Geometry check sheet. Reference: the model listing, model coordinates, mm. A direction names the side the tool comes from. Give positions to 0.01 mm unless a question says otherwise; leave off trailing zeros. Loops run counter-clockwise (first coordinate to the right, second up) from the corner with the lowest first, then second, coordinate; pieces in that order, holes last.
1. Release check for a two-part mould opening along Y. For faces 1 (the cylindrical face through (-1.4, 10.66, 18.24)), 2 (the flat face through (-3.25, -9, 3)), 3 (the flat face through (-1.35, 0, 32)) record: +Y half, -Y half, draft (parallel to the pull), parting line (faces both ways), or undercut.
2. Cross-section at A-A, the plane z = 16.5. Record the cut outline in (x, y).
3. Tool access check on faces 4 (the flat face through (2, 0, 40)), 5 (the flat face through (-2, 0, 25)), 6 (the flat face through (0, -6.5, 32)), 7 (the flat face through (3.25, -9, 3)). Record the directions out of +Z, -Z, +X, -X, +Y, -Y that give a thin tool (end or side, any length) a straight path to the whole face; none if there is none.
4. Go/stop test with flat-tipped pins: pin 1 Ø1 at (x, z) = (-8.5, 28.5) entering from -Y; pin 2 Ø3 at (x, z) = (-8, 6) entering from +Y; pin 3 Ø2.5 at (x, y) = (3, -1.5) entering from -Z. Record where each tip stops, or that it passes through.
5. Cross-section at B-B, the plane z = 4.5. Record the cut outline in (x, y).
6. Material ranges on L1, parallel to X at y = 0, z = 15.75; L2, parallel to Z at x = 2, y = 2.25, recorded low to high.
7. Cross-section at C-C, the plane z = 29. Record the cut outline in (x, y), plus the area to 3 significant figures.
from build123d import *

# Parameters (mm, degrees)
F0_R     = 10.75
F0_R_2   = 7.75
F1_DEPTH = 40
F3_DEPTH = 15
F4_DEPTH = 25
F7_R     = 3
F6_W     = 2.7
F6_H     = 13
F8_DEPTH = 25


# Not quite as in the source:
# - a fillet or chamfer that OpenCascade refuses, or shapes differently, is made with other operations: its cross-section is extruded or revolved along the edge and cut away or added


with BuildPart() as f1:
    # F0 (on Top) → F1 (new body)
    with BuildSketch(Plane.XY):
        Circle(F0_R)
        Circle(F0_R_2, mode=Mode.SUBTRACT)
        Circle(F0_R_2)
    extrude(amount=F1_DEPTH)

    # F2 (on Front) → F3 (cut)
    with BuildSketch(Plane.XZ):
        with BuildLine():
            Line((-3.25, 6), (-3.25, 0))
            Line((-3.25, 0), (3.25, 0))
            Line((3.25, 0), (3.25, 6))
            ThreePointArc((3.25, 6), (0, 9.25), (-3.25, 6))
        make_face()
    extrude(amount=F3_DEPTH, mode=Mode.SUBTRACT)

    # F0 (on Top) → F4 (cut)
    with BuildSketch(Plane.XY):
        Circle(F0_R_2)
    extrude(amount=F4_DEPTH, mode=Mode.SUBTRACT)

    # F7
    f7_edges = [f1.edges().sort_by_distance(p)[0] for p in [
        (-10.75, 0, 40),
    ]]
    fillet(f7_edges, radius=F7_R)

    # F6 (on offset) → F8 (cut)
    with BuildSketch(Plane.XY.offset(40)):
        Rectangle(F6_W, F6_H)
    extrude(amount=-F8_DEPTH, mode=Mode.SUBTRACT)

    # F9: fillet of radius 4 on 1 edges, made by hand


with BuildPart() as f9_tool2:
    # F9_s3 → F9_t4 (revolve)
    with BuildSketch(Plane.XZ):
        with BuildLine():
            ThreePointArc((7.75, 21), (6.5784271247, 23.8284271247), (3.75, 25))
            Line((3.75, 25), (7.75, 25))
            Line((7.75, 25), (7.75, 21))
        make_face()
    revolve(axis=Axis((0, 0, 25), (0, 0, 1)))

    split(bisect_by=Plane.YZ.offset(1.35), keep=Keep.TOP)


with BuildPart() as f1_1:
    add(f1.part)

    # F9_t1: union F9_tool2
    add(f9_tool2.part)


with BuildPart() as f9_tool7:
    # F9_s8 → F9_t9 (revolve)
    with BuildSketch(Plane.XZ):
        with BuildLine():
            ThreePointArc((7.75, 21), (6.5784271247, 23.8284271247), (3.75, 25))
            Line((3.75, 25), (7.75, 25))
            Line((7.75, 25), (7.75, 21))
        make_face()
    revolve(axis=Axis((0, 0, 25), (0, 0, 1)))

    split(bisect_by=Plane.YZ.offset(-1.35), keep=Keep.BOTTOM)


with BuildPart() as f1_2:
    add(f1_1.part)

    # F9_t6: union F9_tool7
    add(f9_tool7.part)


with BuildPart() as f9_tool12:
    # F9_s13 → F9_t14 (revolve)
    with BuildSketch(Plane.XZ):
        with BuildLine():
            ThreePointArc((7.75, 21), (6.5784271247, 23.8284271247), (3.75, 25))
            Line((3.75, 25), (7.75, 25))
            Line((7.75, 25), (7.75, 21))
        make_face()
    revolve(axis=Axis((0, 0, 25), (0, 0, 1)))

    split(bisect_by=Plane.XZ.offset(-6.5), keep=Keep.BOTTOM)


with BuildPart() as f1_3:
    add(f1_2.part)

    # F9_t11: union F9_tool12
    add(f9_tool12.part)


with BuildPart() as f9_tool17:
    # F9_s18 → F9_t19 (revolve)
    with BuildSketch(Plane.XZ):
        with BuildLine():
            ThreePointArc((7.75, 21), (6.5784271247, 23.8284271247), (3.75, 25))
            Line((3.75, 25), (7.75, 25))
            Line((7.75, 25), (7.75, 21))
        make_face()
    revolve(axis=Axis((0, 0, 25), (0, 0, 1)))

    split(bisect_by=Plane.XZ.offset(6.5), keep=Keep.TOP)


with BuildPart() as f1_4:
    add(f1_3.part)

    # F9_t16: union F9_tool17
    add(f9_tool17.part)


solid = f1_4.part
Result:
1. face 1: parting line
1. face 2: draft
1. face 3: undercut
2. outline: circle Ø21.5 at (0, 0); hole circle Ø15.5 at (0, 0)
3. face 4: +Z, +X, -X, +Y, -Y
3. face 5: -Z
3. face 6: +Z, -Z
3. face 7: -Z, -Y
4. pin 1: stops at y = -7.18
4. pin 2: stops at y = 8.56
4. pin 3: stops at z = 24.91
5. outline: (-3.25, -10.25) - (-3.25, -7.04) arc R7.75 cw (long way) to (3.25, -7.04) - (3.25, -10.25) arc R10.75 ccw (long way) to start
6. L1: x = -10.75 to -7.75, 7.75 to 10.75
6. L2: z = 25 to 40
7. outline: circle Ø21.5 at (0, 0); hole (-1.35, -6.5) - (1.35, -6.5) - (1.35, 6.5) - (-1.35, 6.5) - close
7. area: 328 mm2
